from build123d import *

# Parameters (mm, degrees)
F1_DEPTH = 21.8948
F3_DEPTH = 25.4
F4_T     = -2.54
F5_ANGLE = 180


with BuildPart() as f1:
    # F0 (on Front) → F1 (new body)
    with BuildSketch(Plane.XZ):
        Polygon((-50.8, 0), (0, 0), (50.8, 0), (50.8, 38.1), (-50.8, 38.1), align=None)
    extrude(amount=F1_DEPTH)

    # F2 (on Front) → F3 (cut)
    with BuildSketch(Plane.XZ):
        with BuildLine():
            ThreePointArc((-7.874, 24.638), (-10.16, 17.399), (-7.874, 10.16))
            Line((-7.874, 10.16), (-7.874, 0))
            Line((-7.874, 0), (7.874, 0))
            Line((7.874, 0), (7.874, 10.16))
            ThreePointArc((7.874, 10.16), (10.16, 17.399), (7.874, 24.638))
            ThreePointArc((7.874, 24.638), (0, 26.035), (-7.874, 24.638))
        make_face()
    extrude(amount=F3_DEPTH, mode=Mode.SUBTRACT)

    # F4
    f4_openings = [f1.faces().sort_by_distance(p)[0] for p in [
        (29.337, -10.9474, 0),
        (-29.337, -10.9474, 0),
    ]]
    offset(amount=F4_T, openings=f4_openings, kind=Kind.INTERSECTION)


with BuildPart() as f1_1:
    # F5: moved
    add(f1.part.rotate(Axis((50.8, -10.9474, 0), (0, 1, 0)), F5_ANGLE))


solid = f1_1.part
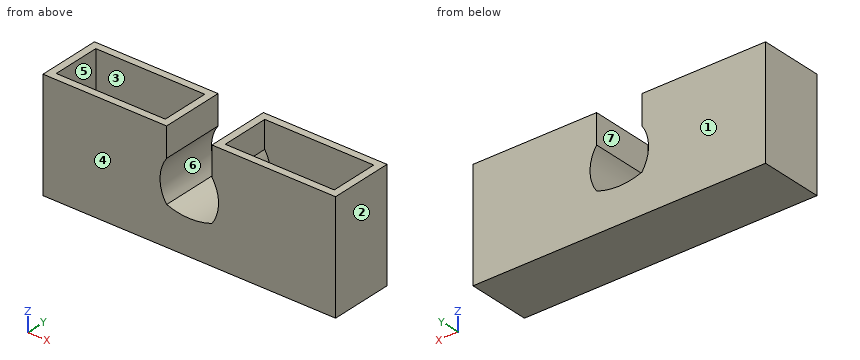
The model under review builds one solid part; all positions refer to its coordinate system, in mm. Face numbers are marked on the shaded views. A direction names the side the tool comes from. Round coordinates to 2 decimals unless told otherwise and drop trailing zeros. Loops run counter-clockwise (first coordinate to the right, second up) from the corner with the lowest first, then second, coordinate; pieces in that order, holes last. Notation, with made-up numbers: (58.25, -36.75) - (68.25, -36.75) arc R37 ccw to (68.25, 2.25) - close; hole circle Ø9 at (-24.5, 46). An arc over 180 degrees is marked (long way). Use CSV: the item, a comma, the result in double quotes.
(1) Machinability: for the marked faces 4, 5, 6 and 7, which of the approach directions +Z, -Z, +X, -X, +Y, -Y give a long, thin tool a straight path to every point of the face, cutting with its end or side? Answer none if there is none.
Working result:
face 4,"+Z, -Z, +X, -X, -Y"
face 5,"+Z"
face 6,"+Y, -Y"
face 7,"+Z, +Y, -Y"
(2) Clearance check with a flat-ended pin moving along its axis: P1, Ø12, axis at x = 103, z = -10.5, coming from the +Y side. State where the tip first meets the part, or that it passes through.
Working result:
P1,"passes through"
(3) Take a section at D-D, the plane z = -20. Give the boundary of the cut face in (x, y).
Working result:
outline,"(50.8, -21.89) - (91.71, -21.89) - (91.71, 0) - (50.8, 0) - close; (111.49, -21.89) - (152.4, -21.89) - (152.4, 0) - (111.49, 0) - close; hole (53.34, -19.35) - (89.13, -19.35) - (89.13, -2.54) - (53.34, -2.54) - close; hole (114.07, -19.35) - (149.86, -19.35) - (149.86, -2.54) - (114.07, -2.54) - close"
(4) Take a section at C-C, the plane x = 141. Give the boundary of the cut face in (y, z).
Working result:
outline,"(-21.89, -38.1) - (0, -38.1) - (0, 0) - (-2.54, 0) - (-2.54, -35.56) - (-19.35, -35.56) - (-19.35, 0) - (-21.89, 0) - close"
(5) The part is to be moulded in two halves that separate along Y. For the marked faces 1, 2 and 3, say which applies: pulls with the +Y half, pulls with the -Y half, needs draft (parallel to the pull), parting line crosses it, or undercut.
Working result:
face 1,"pulls with the +Y half"
face 2,"needs draft"
face 3,"undercut"
(6) Take a section at A-A, the plane y = -10.25. Give the boundary of the cut face in (x, z).
Working result:
outline,"(50.8, -38.1) - (152.4, -38.1) - (152.4, 0) - (149.86, 0) - (149.86, -35.56) - (53.34, -35.56) - (53.34, 0) - (50.8, 0) - close; (91.19, -9.4) arc R15.14 ccw to (92.13, -26.74) arc R25.43 ccw to (111.07, -26.74) arc R15.14 ccw to (112.01, -9.4) - (112.01, 0) - (109.47, 0) - (109.47, -10.16) arc R12.6 cw to (109.47, -24.64) arc R22.89 cw to (93.73, -24.64) arc R12.6 cw to (93.73, -10.16) - (93.73, 0) - (91.19, 0) - close"
(7) For line 1 (X direction, y = -4.25, z = -6.5); line 2 (Y direction, x = 100.5, z = -33.5); line 3 (X direction, y = -9.5, z = -15), list the stretches that pass through material, from the lowest coordinate up.
Working result:
line 1,"x = 50.8 to 53.34, 91.19 to 93.73, 109.47 to 112.01, 149.86 to 152.4"
line 2,"y = -21.89 to -19.35, -2.54 to 0"
line 3,"x = 50.8 to 53.34, 89.09 to 91.67, 111.53 to 114.11, 149.86 to 152.4"
(8) Take a section at B-B, the plane z = -16. Give the boundary of the cut face in (x, y).
Working result:
outline,"(50.8, -21.89) - (91.52, -21.89) - (91.52, 0) - (50.8, 0) - close; (111.68, -21.89) - (152.4, -21.89) - (152.4, 0) - (111.68, 0) - close; hole (53.34, -19.35) - (88.96, -19.35) - (88.96, -2.54) - (53.34, -2.54) - close; hole (114.24, -19.35) - (149.86, -19.35) - (149.86, -2.54) - (114.24, -2.54) - close"
